Verification items for the finished model (mm, model axes). Face numbers are marked on the shaded views. A direction names the side the tool comes from. Round coordinates to 2 decimals unless told otherwise and drop trailing zeros. Loops run counter-clockwise (first coordinate to the right, second up) from the corner with the lowest first, then second, coordinate; pieces in that order, holes last. Notation, with made-up numbers: M 35,80 L 86,80 A27 cw 86,101 Z; hole C -31,-6 d9. An arc over 180 degrees is marked long. Write item = value, one per line. Start each with the question number.
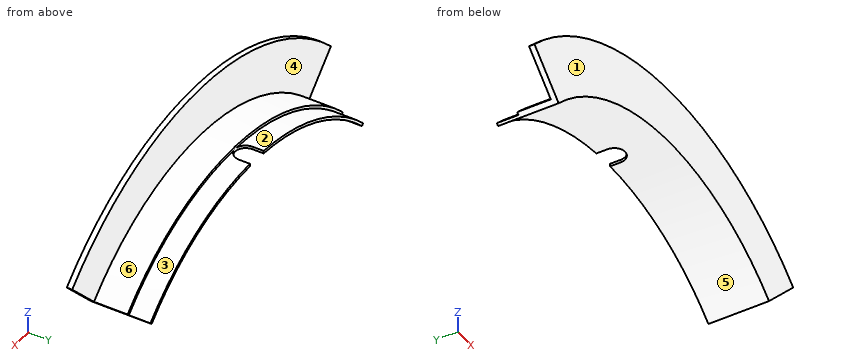
Autodesk Inventor part; units mm, degrees
ref_plane "YZ Plane" through (0, 0, 0) normal (1, 0, 0) x (0, 1, 0)
ref_plane "XZ Plane" through (0, 0, 0) normal (0, 1, 0) x (-1, 0, 0)
ref_plane "XY Plane" through (0, 0, 0) normal (0, 0, 1) x (1, 0, 0)
sketch "Sketch1" plane through (0, 0, 0) normal (1, 0, 0) x (0, 1, 0)
  line L0 (0, 0) -> (50.8, 0)
  line L1 (0, 138.1125) -> (26.719, 138.1125)
  line L2 (0, 138.1125) -> (0, 169.8625)
  line L3 (0, 169.8625) -> (3.175, 169.8625)
  line L4 (3.175, 169.8625) -> (3.175, 141.2875)
  line L5 (3.175, 141.2875) -> (22.9489, 141.2875)
  line L6 (60.325, 141.2875) -> (60.325, 179.3875)
  line L7 (60.325, 179.3875) -> (63.5, 179.3875)
  line L8 (63.5, 179.3875) -> (63.5, 138.1125)
  line L9 (35.6489, 138.1125) -> (26.719, 138.1125)
  line L10 (29.2989, 139.7) -> (22.9489, 139.7)
  line L11 (22.9489, 139.7) -> (22.9489, 141.2875)
  line L12 (29.2989, 139.7) -> (35.6489, 139.7)
  line L13 (35.6489, 139.7) -> (35.6489, 138.1125)
  line L14 (29.2989, 166.1379) -> (29.2989, 141.2875)
  line L15 (29.2989, 138.1125) -> (29.2989, 120.1049)
  point P0 (62.1333, 179.3875)
  point P1 (1.5875, 169.8625)
  dimension "d0" = 50.8
  dimension "d1" = 138.1125
  dimension "d2" = 31.75
  dimension "d3" = 3.175
  dimension "d4" = 3.175
  dimension "d5" = 57.15
  dimension "d6" = 38.1
  dimension "d7" = 3.175
  dimension "d13" = 26.1239
  dimension "d14" = 1.5875
  dimension "d15" = 6.35
  dimension "d16" = 6.35
revolve "Revolution1" add sketch "Sketch1" angle 360 about axis through (0, 0, 0) along (0, 1, 0)
ref_plane "Work Plane2" through (0, 1.5875, 169.8625) normal (0, 0, 1) x (1, 0, 0)
sketch "Sketch3" plane through (0, 1.5875, 169.8625) normal (0, 0, 1) x (1, 0, 0)
  arc A0 (-6.3749, 27.6865) -> (6.3749, 27.6865) centre (0, 27.6865) ccw
  line L0 (138.1125, 34.0614) -> (-138.1125, 34.0614)
  line L1 (-6.3749, 27.6865) -> (-6.3749, 34.0614)
  line L2 (6.3749, 27.6865) -> (6.3749, 34.0614)
  point P0 (0, -1.5875)
  point P1 (0, 17.4621)
extrude "Extrusion2" cut sketch "Sketch3" against normal through all
sketch "Sketch4" plane through (0, 0, 0) normal (0, -1, 0) x (1, 0, 0)
  line L0 (0, 0) -> (-198.1259, 198.1259)
  line L1 (0, 0) -> (280.1923, 0) construction
  line L2 (-198.1259, 198.1259) -> (-198.1259, -227.7187)
  line L3 (-198.1259, -227.7187) -> (214.1573, -227.7187)
  line L4 (0, 0) -> (198.1259, 198.1259)
  line L5 (198.1259, 198.1259) -> (214.1573, -227.7187)
  dimension "d19" = 135
  dimension "d20" = 90
extrude "Extrusion3" cut sketch "Sketch4" against normal through all
properties part number "Layer2_Bottom_Quarter"
1. Section check B-B, the plane y = 16. Enter the section's corners in (x, z) (1 decimal), and give its area (3 significant figures).
2. Mould release check, pull along X, two halves, no side actions. Record for the marked faces 4, 5 and 6: pulls with the +X half, pulls with the -X half, needs draft (parallel to the pull), parting line crosses it, or undercut.
3. Section check D-D, the plane x = -73.5. Enter the section's corners in (y, z) (3 decimals), and give its area (3 significant figures).
4. Section check A-A, the plane x = -37.5. Enter the section's corners in (y, z) (3 decimals), and give its area (3 significant figures).
5. Tool access check on the marked faces 1, 2 and 3. Record the directions out of +Z, -Z, +X, -X, +Y, -Y that give a thin tool (end or side, any length) a straight path to the whole face; none if there is none.
6. Gauge pin test, flat ends, axial feed: P1, Ø1, axis at y = 7, z = 115, coming from the +X side; P2, Ø21, axis at x = 35, z = 149.5, coming from the +Y side (3 decimals); P3, Ø10, axis at y = 4, z = 157.5, coming from the +X side. Record the tip position at first contact, or that the pin passes through.
7. Section check C-C, the plane z = 158.5. Enter the section's corners in (x, y) (3 decimals), and give its area (3 significant figures).
8. Thickness scan on line 1 (Y direction, x = -5.5, z = 148.5) (3 decimals); line 2 (Z direction, x = -7, y = 26) (3 decimals); line 3 (X direction, y = 28.5, z = 121). Record the ranges inside material, lowest first.
Computed values:
q1.outline = M -99.9,99.9 L -97.7,97.7 A138.1 cw 97.7,97.7 L 99.9,99.9 A141.3 ccw Z
q1.area = 697 mm2
q2.face_4 = needs draft
q2.face_5 = undercut
q2.face_6 = parting line crosses it
q3.outline = M 0,116.931 L 35.649,116.931 L 35.649,118.802 L 22.949,118.802 L 22.949,120.664 L 3.175,120.664 L 3.175,153.137 L 0,153.137 Z
q3.area = 213 mm2
q4.outline = M 0,132.924 L 35.649,132.924 L 35.649,134.573 L 22.949,134.573 L 22.949,136.22 L 3.175,136.22 L 3.175,165.671 L 0,165.671 Z
q4.area = 190 mm2
q5.face_1 = +Z, -Z, +X, -X, -Y
q5.face_2 = +Z, -X, +Y
q5.face_3 = +Z, +X, +Y
q6.P1 = 82.78
q6.P2 = 3.175
q6.P3 = 74.67
q7.outline = M -61.082,0 L 61.082,0 L 61.082,3.175 L -61.082,3.175 Z
q7.area = 388 mm2
q8.line_1 = 0 to 3.175
q8.line_2 = 137.935 to 139.525
q8.line_3 = -69.82 to -66.59, 66.59 to 69.82
